Geometry check sheet. Reference: the model listing, model coordinates, mm. A direction names the side the tool comes from. Round coordinates to 2 decimals unless told otherwise and drop trailing zeros. Write each loop counter-clockwise with the first axis right and the second up, starting at its lowest first coordinate (ties: lowest second). Pieces come first, ordered by that corner, then holes. Notation, with made-up numbers: (-35, -20) - (24, -20) arc R6 cw to (24, -15) - close; hole circle Ø7 at (70.25, -35.5). An arc over 180 degrees is marked (long way). One line per question, with ' | ' between items. Start each with the question number.
from build123d import *

# Parameters (mm, degrees)
EXTRUDE_1_DEPTH      = 4
EXTRUDE_2_DEPTH      = 0.4
CHAMFER_1_SIZE       = 1
FILLET_1_R           = 1
EXTRUDE_3_DEPTH      = 10
EXTRUDE_3_DEPTH_BACK = 10
SKETCH_3_R           = 2.2
EXTRUDE_4_DEPTH      = 0.8
FILLET_2_R           = 0.4


with BuildPart() as part:
    # 草图1 → 凸台-拉伸1 (new body)
    with BuildSketch(Plane(origin=(0, 0, 0), x_dir=(1, 0, 0), z_dir=(0, 1, 0))):
        with BuildLine():
            Line((-12.529964086, 13.2), (12.529964086, 13.2))
            ThreePointArc((12.529964086, 13.2), (18.2, 0), (12.529964086, -13.2))
            Line((12.529964086, -13.2), (-12.529964086, -13.2))
            ThreePointArc((-12.529964086, -13.2), (-18.2, 0), (-12.529964086, 13.2))
        make_face()
        with BuildLine():
            Line((-12.124355653, 12.2), (12.124355653, 12.2))
            ThreePointArc((12.124355653, 12.2), (17.2, 0), (12.124355653, -12.2))
            Line((12.124355653, -12.2), (-12.124355653, -12.2))
            ThreePointArc((-12.124355653, -12.2), (-17.2, 0), (-12.124355653, 12.2))
        make_face(mode=Mode.SUBTRACT)
    extrude(amount=EXTRUDE_1_DEPTH)

    # 草图2 → 凸台-拉伸2 (add)
    with BuildSketch(Plane.XZ):
        with BuildLine():
            Line((-12.124355653, -12.2), (-9, -12.2))
            Line((-9, -12.2), (-9, -11.2))
            Line((-9, -11.2), (-11.704699911, -11.2))
            ThreePointArc((-11.704699911, -11.2), (-12.433722739, -10.384726228), (-13.106075309, -9.522121087))
            Line((-13.106075309, -9.522121087), (-13.915092303, -10.109906339))
            ThreePointArc((-13.915092303, -10.109906339), (-13.061597733, -11.190829489), (-12.124355653, -12.2))
        make_face()
        with BuildLine():
            Line((9, -12.2), (12.124355653, -12.2))
            ThreePointArc((12.124355653, -12.2), (13.061597733, -11.190829489), (13.915092303, -10.109906339))
            Line((13.915092303, -10.109906339), (13.106075309, -9.522121087))
            ThreePointArc((13.106075309, -9.522121087), (12.433722739, -10.384726228), (11.704699911, -11.2))
            Line((11.704699911, -11.2), (9, -11.2))
            Line((9, -11.2), (9, -12.2))
        make_face()
        with BuildLine():
            Line((13.106075309, 9.522121087), (13.915092303, 10.109906339))
            ThreePointArc((13.915092303, 10.109906339), (13.061597733, 11.190829489), (12.124355653, 12.2))
            Line((12.124355653, 12.2), (9, 12.2))
            Line((9, 12.2), (9, 11.2))
            Line((9, 11.2), (11.704699911, 11.2))
            ThreePointArc((11.704699911, 11.2), (12.433722739, 10.384726228), (13.106075309, 9.522121087))
        make_face()
        with BuildLine():
            ThreePointArc((-12.124355653, 12.2), (-13.061597733, 11.190829489), (-13.915092303, 10.109906339))
            Line((-13.915092303, 10.109906339), (-13.106075309, 9.522121087))
            ThreePointArc((-13.106075309, 9.522121087), (-12.433722739, 10.384726228), (-11.704699911, 11.2))
            Line((-11.704699911, 11.2), (-9, 11.2))
            Line((-9, 11.2), (-9, 12.2))
            Line((-9, 12.2), (-12.124355653, 12.2))
        make_face()
    extrude(amount=-EXTRUDE_2_DEPTH)

    # 倒角1
    # the kernel refuses this chamfer: 1 mm, written as the material it adds along each edge
    with BuildSketch(Plane(origin=(9, 0, -12.2), x_dir=(-1, 0, 0), z_dir=(0, 1, 0))) as chamfer_1_piece_1_section:
        Polygon((CHAMFER_1_SIZE, 0), (0, CHAMFER_1_SIZE), (0, 0), align=None)
    chamfer_1_piece_1 = extrude(amount=0.4, mode=Mode.PRIVATE)
    chamfer_1_piece_1 = split(chamfer_1_piece_1, bisect_by=Plane(origin=(9, 0, -11.2), z_dir=(0, 0, -1)), keep=Keep.TOP, mode=Mode.PRIVATE)
    add(chamfer_1_piece_1)
    with BuildSketch(Plane(origin=(13.915092303, 0, -10.109906339), x_dir=(0.5646701289866782, 0, 0.8253166940212516), z_dir=(0, 1, 0))) as chamfer_1_piece_2_section:
        with BuildLine():
            Line((0.972875022, 0), (CHAMFER_1_SIZE * 0.0282812506504, -CHAMFER_1_SIZE * 0.999600005433))
            Line((CHAMFER_1_SIZE * 0.0282812506504, -CHAMFER_1_SIZE * 0.999600005433), (0, 0))
            ThreePointArc((0, 0), (0.500167916, 0.006874426), (0.972875022, 0))
        make_face()
    chamfer_1_piece_2 = extrude(amount=0.4, mode=Mode.PRIVATE)
    chamfer_1_piece_2 = chamfer_1_piece_2 - Plane(origin=(0, 0, 0), x_dir=(0.8090169943749429, 0, -0.5877852522924794), z_dir=(0, -1, 0)) * Cylinder(16.2, 5, mode=Mode.PRIVATE)
    add(chamfer_1_piece_2)
    with BuildSketch(Plane(origin=(13.915092303, 0, 10.109906339), x_dir=(0.5646701289866733, 0, -0.825316694021255), z_dir=(0, 1, 0))) as chamfer_1_piece_3_section:
        with BuildLine():
            Line((0.972875022, 0), (CHAMFER_1_SIZE * 0.0282812506504, CHAMFER_1_SIZE * 0.999600005433))
            Line((CHAMFER_1_SIZE * 0.0282812506504, CHAMFER_1_SIZE * 0.999600005433), (0, 0))
            ThreePointArc((0, 0), (0.500167916, -0.006874426), (0.972875022, 0))
        make_face()
    chamfer_1_piece_3 = extrude(amount=0.4, mode=Mode.PRIVATE)
    chamfer_1_piece_3 = chamfer_1_piece_3 - Plane(origin=(0, 0, 0), x_dir=(0.7225123401678771, 0, 0.6913580246913591), z_dir=(0, -1, 0)) * Cylinder(16.2, 5, mode=Mode.PRIVATE)
    add(chamfer_1_piece_3)
    with BuildSketch(Plane(origin=(9, 0, 12.2), x_dir=(-1, 0, 0), z_dir=(0, 1, 0))) as chamfer_1_piece_4_section:
        Polygon((CHAMFER_1_SIZE, 0), (0, -CHAMFER_1_SIZE), (0, 0), align=None)
    chamfer_1_piece_4 = extrude(amount=0.4, mode=Mode.PRIVATE)
    chamfer_1_piece_4 = split(chamfer_1_piece_4, bisect_by=Plane(origin=(9, 0, 11.2), z_dir=(0, 0, 1)), keep=Keep.TOP, mode=Mode.PRIVATE)
    add(chamfer_1_piece_4)
    with BuildSketch(Plane(origin=(-9, 0, 12.2), x_dir=(1, 0, 0), z_dir=(0, 1, 0))) as chamfer_1_piece_5_section:
        Polygon((CHAMFER_1_SIZE, 0), (0, CHAMFER_1_SIZE), (0, 0), align=None)
    chamfer_1_piece_5 = extrude(amount=0.4, mode=Mode.PRIVATE)
    chamfer_1_piece_5 = split(chamfer_1_piece_5, bisect_by=Plane(origin=(-9, 0, 11.2), z_dir=(0, 0, 1)), keep=Keep.TOP, mode=Mode.PRIVATE)
    add(chamfer_1_piece_5)
    with BuildSketch(Plane(origin=(-13.915092303, 0, 10.109906339), x_dir=(-0.5646701289866741, 0, -0.8253166940212543), z_dir=(0, 1, 0))) as chamfer_1_piece_6_section:
        with BuildLine():
            Line((0.972875022, 0), (CHAMFER_1_SIZE * 0.0282812506504, -CHAMFER_1_SIZE * 0.999600005433))
            Line((CHAMFER_1_SIZE * 0.0282812506504, -CHAMFER_1_SIZE * 0.999600005433), (0, 0))
            ThreePointArc((0, 0), (0.500167916, 0.006874426), (0.972875022, 0))
        make_face()
    chamfer_1_piece_6 = extrude(amount=0.4, mode=Mode.PRIVATE)
    chamfer_1_piece_6 = chamfer_1_piece_6 - Plane(origin=(0, 0, 0), x_dir=(-0.809016994374947, 0, 0.5877852522924738), z_dir=(0, -1, 0)) * Cylinder(16.2, 5, mode=Mode.PRIVATE)
    add(chamfer_1_piece_6)
    with BuildSketch(Plane(origin=(-13.915092303, 0, -10.109906339), x_dir=(-0.5646701289866836, 0, 0.8253166940212479), z_dir=(0, 1, 0))) as chamfer_1_piece_7_section:
        with BuildLine():
            Line((0.972875022, 0), (CHAMFER_1_SIZE * 0.0282812506504, CHAMFER_1_SIZE * 0.999600005433))
            Line((CHAMFER_1_SIZE * 0.0282812506504, CHAMFER_1_SIZE * 0.999600005433), (0, 0))
            ThreePointArc((0, 0), (0.500167916, -0.006874426), (0.972875022, 0))
        make_face()
    chamfer_1_piece_7 = extrude(amount=0.4, mode=Mode.PRIVATE)
    chamfer_1_piece_7 = chamfer_1_piece_7 - Plane(origin=(0, 0, 0), x_dir=(-0.7225123401678729, 0, -0.6913580246913635), z_dir=(0, -1, 0)) * Cylinder(16.2, 5, mode=Mode.PRIVATE)
    add(chamfer_1_piece_7)
    with BuildSketch(Plane(origin=(-9, 0, -12.2), x_dir=(1, 0, 0), z_dir=(0, 1, 0))) as chamfer_1_piece_8_section:
        Polygon((CHAMFER_1_SIZE, 0), (0, -CHAMFER_1_SIZE), (0, 0), align=None)
    chamfer_1_piece_8 = extrude(amount=0.4, mode=Mode.PRIVATE)
    chamfer_1_piece_8 = split(chamfer_1_piece_8, bisect_by=Plane(origin=(-9, 0, -11.2), z_dir=(0, 0, -1)), keep=Keep.TOP, mode=Mode.PRIVATE)
    add(chamfer_1_piece_8)

    # 圆角1
    fillet_1_edges = [part.edges().sort_by_distance(p)[0] for p in [
        (-8, 0.2, -12.2),
        (8, 0.2, -12.2),
        (14.464445768, 0.2, 9.306976342),
        (14.464445768, 0.2, -9.306976342),
        (-8, 0.2, 12.2),
        (8, 0.2, 12.2),
        (-14.464445768, 0.2, -9.306976342),
        (-14.464445768, 0.2, 9.306976342),
        (-11.704699911, 0.2, -11.2),
        (-9, 0.2, -11.2),
        (-13.106075309, 0.2, -9.522121087),
        (11.704699911, 0.2, -11.2),
        (13.106075309, 0.2, -9.522121087),
        (9, 0.2, -11.2),
        (11.704699911, 0.2, 11.2),
        (9, 0.2, 11.2),
        (13.106075309, 0.2, 9.522121087),
        (-11.704699911, 0.2, 11.2),
        (-13.106075309, 0.2, 9.522121087),
        (-9, 0.2, 11.2),
    ]]
    fillet(fillet_1_edges, radius=FILLET_1_R)

    # 草图3 → 凸台-拉伸3 (add, two sides: drawn at the far end of the back side and taken through both)
    with BuildSketch(Plane(origin=(0, 0, 0), x_dir=(0, 0, -1), z_dir=(1, 0, 0)).offset(-EXTRUDE_3_DEPTH_BACK)):
        with BuildLine():
            Line((-18, 0), (-13.2, 0))
            Line((-13.2, 0), (-13.2, 4))
            Line((-13.2, 4), (-13.2, 6.4))
            ThreePointArc((-13.2, 6.4), (-22, 8), (-18, 0))
        make_face()
        with Locations((-18, 5)):
            Circle(SKETCH_3_R, mode=Mode.SUBTRACT)
    extrude(amount=EXTRUDE_3_DEPTH + EXTRUDE_3_DEPTH_BACK)

    # 草图4 → 凸台-拉伸4 (add)
    with BuildSketch(Plane.XZ):
        with BuildLine():
            Line((16.076069171, 2), (17.083325203, 2))
            ThreePointArc((17.083325203, 2), (17.2, 0), (17.083325203, -2))
            Line((17.083325203, -2), (16.076069171, -2))
            ThreePointArc((16.076069171, -2), (16.2, 0), (16.076069171, 2))
        make_face()
        with BuildLine():
            Line((-16.076069171, 2), (-17.083325203, 2))
            ThreePointArc((-17.083325203, 2), (-17.2, 0), (-17.083325203, -2))
            Line((-17.083325203, -2), (-16.076069171, -2))
            ThreePointArc((-16.076069171, -2), (-16.2, 0), (-16.076069171, 2))
        make_face()
    extrude(amount=-EXTRUDE_4_DEPTH)

    # 圆角2
    fillet_2_edges = [part.edges().sort_by_distance(p)[0] for p in [
        (17.083325203, 0.4, 2),
        (17.083325203, 0.4, -2),
        (16.076069171, 0.4, -2),
        (16.076069171, 0.4, 2),
        (-16.076069171, 0.4, 2),
        (-16.076069171, 0.4, -2),
        (-17.083325203, 0.4, -2),
        (-17.083325203, 0.4, 2),
    ]]
    fillet(fillet_2_edges, radius=FILLET_2_R)


solid = part.part
Q1. Set-up check for faces 5 (the flat face through (-1, 0, 13)), 6 (the flat face through (11.7, 0.4, 11.3)), 7 (the cylindrical face through (-12.445, 0.197, -10.371)): record each of +Z, -Z, +X, -X, +Y, -Y from which the full face is reachable in a straight line by a thin tool's end or side.
Q2. Section check C-C, the plane y = 8.5. Record the cut outline in (x, z), then the cut area to 3 significant figures.
Q3. Go/stop test with flat-tipped pins: P1, Ø3, axis at y = 2.5, z = 18.5, coming from the +X side; P2, Ø0.8, axis at x = 11, y = 1.5, coming from the +Z side; P3, Ø5, axis at y = 4, z = 3, coming from the +X side. Record where each tip stops, or that it passes through.
Q4. Draft check along Z on faces 1 (the cylindrical face through (-12.457, 0.197, 10.357)), 2 (the flat face through (10, 2.8, 17.1)), 3 (the cylindrical face through (-18.2, 2, 0.2)), 4 (the cylindrical face through (12.445, 0.197, 10.371)). Enter one of: pulls with the +Z half, pulls with the -Z half, needs draft (parallel to the pull), parting line crosses it, or undercut.
Q5. Section check A-A, the plane y = 5. Record the cut outline in (x, z).
Q6. Thickness scan on line 1 (Z direction, x = 1.5, y = 3); line 2 (Z direction, x = -6.5, y = 3.5); line 3 (Y direction, x = -2.25, z = 18). Record the ranges inside material, lowest first.
Q7. Section check B-B, the plane z = 8. Record the cut outline in (x, y).
Result sheet:
1) face 5: +Z, -Z, +X, -X, -Y | face 6: +Y | face 7: +Y, -Y
2) outline: (-10, 14.43) - (10, 14.43) - (10, 21.57) - (-10, 21.57) - close | area: 143 mm²
3) P1: x = 10 | P2: z = 13.2 | P3: x = 18.19
4) face 1: undercut | face 2: needs draft | face 3: parting line crosses it | face 4: undercut
5) outline: (-10, 13.2) - (10, 13.2) - (10, 15.8) - (-10, 15.8) - close; (-10, 20.2) - (10, 20.2) - (10, 23) - (-10, 23) - close
6) line 1: -13.2 to -12.2, 12.2 to 17.08, 18.92 to 22.58 | line 2: -13.2 to -12.2, 12.2 to 16.39, 19.61 to 22.77 | line 3: 0 to 2.8, 7.2 to 10
7) outline: (-16.35, 0) - (-15.23, 0) - (-15.23, 4) - (-16.35, 4) - close; (15.23, 0) - (16.35, 0) - (16.35, 4) - (15.23, 4) - close
